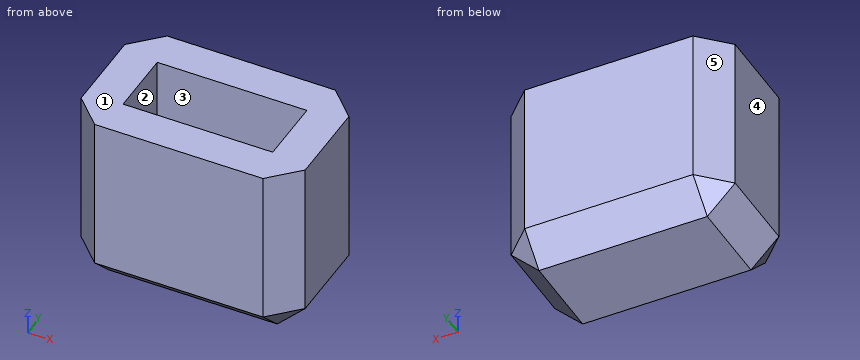
```python
from build123d import *

# Parameters (mm, degrees)
SKETCH1_W           = 12.04
SKETCH1_H           = 7.58
SKETCH1_W_2         = 8.04
SKETCH1_H_2         = 3.58
BOSS_EXTRUDE1_DEPTH = 8
SKETCH1_2_W         = 12.04
SKETCH1_2_H         = 7.58
SKETCH1_2_W_2       = 8.04
SKETCH1_2_H_2       = 3.58
BOSS_EXTRUDE2_DEPTH = 2
CHAMFER1_SIZE       = 1.5


with BuildPart() as part:
    # Sketch1 → Boss-Extrude1 (new body)
    with BuildSketch(Plane.XY):
        Rectangle(SKETCH1_W, SKETCH1_H)
        Rectangle(SKETCH1_W_2, SKETCH1_H_2, mode=Mode.SUBTRACT)
    extrude(amount=BOSS_EXTRUDE1_DEPTH)

    # Sketch1<2> → Boss-Extrude2 (add)
    # profile 1 of 2: a face of its own
    with BuildSketch(Plane.XY):
        Rectangle(SKETCH1_2_W, SKETCH1_2_H)
        Rectangle(SKETCH1_2_W_2, SKETCH1_2_H_2, mode=Mode.SUBTRACT)
    # profile 2 of 2: a face of its own
    with BuildSketch(Plane.XY):
        Rectangle(SKETCH1_2_W_2, SKETCH1_2_H_2)
    extrude(amount=-BOSS_EXTRUDE2_DEPTH)

    # Chamfer1
    chamfer1_edges = [part.edges().sort_by_distance(p)[0] for p in [
        (0, -3.79, -2),
        (-6.02, 0, -2),
        (6.02, 0, -2),
        (0, 3.79, -2),
        (6.02, -3.79, 3),
        (-6.02, -3.79, 3),
        (-6.02, 3.79, 3),
        (6.02, 3.79, 3),
    ]]
    chamfer(chamfer1_edges, length=CHAMFER1_SIZE)


solid = part.part
```
The model under review builds one solid part; all positions refer to its coordinate system, in mm. Face numbers are marked on the shaded views. A direction names the side the tool comes from. Round coordinates to 2 decimals unless told otherwise and drop trailing zeros. Loops run counter-clockwise (first coordinate to the right, second up) from the corner with the lowest first, then second, coordinate; pieces in that order, holes last. Notation, with made-up numbers: (32, 62.25) -> (73, 62.25) arc R37 ccw to (73, 99.25) -> close; hole circle Ø7 at (87, -21). An arc over 180 degrees is marked (long way). Answer as a JSON object with one key per item and string values. Group by question number.
1) For pin 1 Ø4 at (y, z) = (-3, 6.5) entering from +X; pin 2 Ø1.1 at (x, y) = (2, -0.5) entering from +Z, all flat-tipped, find the tip position at first contact; note any pin that passes through.
2) We need section C-C on y = -1. Write out the cut boundary in (x, z).
3) Mouldability with a two-part tool opening along Y and no side actions: class the marked faces 3, 4 and 5 as released by +Y, released by -Y, zero draft, split by the parting line, or undercut.
4) We need section D-D on z = -0.75. Write out the cut boundary in (x, y), then the cut area to 3 significant figures.
5) We need section B-B on x = 0. Write out the cut boundary in (y, z).
6) We need section A-A on z = 6.25. Write out the cut boundary in (x, y), then the cut area to 3 significant figures.
7) For line 1 (Y direction, x = -3, z = 7); line 2 (X direction, y = 0, z = 1.25); line 3 (Z direction, x = 1.5, y = 1), list the stretches that pass through material, from the lowest coordinate up. Write a range as [from, to].
8) For the marked faces 1 and 2, list the 3-axis set-ups (+Z, -Z, +X, -X, +Y, -Y) from which the entire face can be reached by the end or side of a thin tool; tool diameter is ignored.
Result set:
{
 "1": {"pin 1": "x = 6.02", "pin 2": "z = 0"},
 "2": {"outline": "(-6.02, -0.5) -> (-4.52, -2) -> (4.52, -2) -> (6.02, -0.5) -> (6.02, 8) -> (4.02, 8) -> (4.02, 0) -> (-4.02, 0) -> (-4.02, 8) -> (-6.02, 8) -> close"},
 "3": {"face 3": "undercut", "face 4": "zero draft", "face 5": "released by +Y"},
 "4": {"outline": "(-5.77, -2.29) -> (-4.52, -3.54) -> (4.52, -3.54) -> (5.77, -2.29) -> (5.77, 2.29) -> (4.52, 3.54) -> (-4.52, 3.54) -> (-5.77, 2.29) -> close", "area": "78.6 mm²"},
 "5": {"outline": "(-3.79, -0.5) -> (-2.29, -2) -> (2.29, -2) -> (3.79, -0.5) -> (3.79, 8) -> (1.79, 8) -> (1.79, 0) -> (-1.79, 0) -> (-1.79, 8) -> (-3.79, 8) -> close"},
 "6": {"outline": "(-6.02, -2.29) -> (-4.52, -3.79) -> (4.52, -3.79) -> (6.02, -2.29) -> (6.02, 2.29) -> (4.52, 3.79) -> (-4.52, 3.79) -> (-6.02, 2.29) -> close; hole (-4.02, -1.79) -> (4.02, -1.79) -> (4.02, 1.79) -> (-4.02, 1.79) -> close", "area": "58.0 mm²"},
 "7": {"line 1": "[-3.79, -1.79], [1.79, 3.79]", "line 2": "[-6.02, -4.02], [4.02, 6.02]", "line 3": "[-2, 0]"},
 "8": {"face 1": "+Z, +X, -X, +Y, -Y", "face 2": "+Z"}
}
